Input: part model. Units: mm. Frame: model coordinates. Face numbers are marked on the shaded views. A direction names the side the tool comes from. Coordinates: 2 decimals unless noted, no trailing zeros. Order: outer loops, then holes, each group sorted by start corner. A loop starts at its lowest first (then second) coordinate and runs counter-clockwise, first axis right, second up. Notation, with made-up numbers: (8.25, 11) - (25.25, 11) arc R13 ccw to (25.25, 36) - close; hole circle Ø1 at (43, 22.5). An arc over 180 degrees is marked (long way). Answer as CSV lines item,"result". Start each with the question number.
Item 1: Draft query along Z for the marked faces 1, 2 and 3. Return one class per face: +Z half, -Z half, draft (parallel to the pull), parting line (faces both ways), or undercut.
Item 2: Section C-C (z = 14.25). Output: boundary loops of the cut face in (x, y), and give its area (3 significant figures).
Item 3: First-contact query: pin 1 (6 mm diameter, centred on x = -2, z = 11, fed in from -Y); pin 2 (1.6 mm diameter, centred on x = -3.5, z = 10.5, fed in from +Y); pin 3 (10 mm diameter, centred on y = 6, z = 9, fed in from -X); pin 4 (1.6 mm diameter, centred on x = -5, z = 10, fed in from -Y). Flat tips, straight axial feed; report the tip coordinate or a pass-through.
Item 4: Material intervals for line 1 along Z through (x, y) = (-3.25, 2.5); line 2 along Y through (x, z) = (-6.25, 10.5); line 3 along Z through (x, y) = (-6.5, 0.5), sorted ascending.
Item 5: Access query for the marked faces 4 and 5. Directions: +Z, -Z, +X, -X, +Y, -Y. A direction counts if a zero-diameter tool reaches every point of the face in a straight line with its end or side. Return the directions, or none.
Item 6: Section A-A (z = 9.75). Output: boundary loops of the cut face in (x, y).
Item 7: Section B-B (z = 7.5). Output: boundary loops of the cut face in (x, y), and give its area (3 significant figures).
Autodesk Fusion 360 part; units mm, degrees
sketch "Sketch1" plane through (0, 0, 0) normal (0, 0, 1) x (1, 0, 0)
  line L0 (0, 10) -> (0, -10)
  arc A0 (0, 10) -> (0, -10) centre (0, 0) ccw
extrude "Extrude1" add sketch "Sketch1" along normal blind 20
sketch "Sketch2" plane through (0, 0, 0) normal (1, 0, 0) x (0, 0, -1)
  line L0 (0, -10) -> (0, 10)
  line L1 (0, 10) -> (-20, 10)
  line L2 (-20, 10) -> (-20, -10)
  line L3 (-20, -10) -> (0, -10)
  line L4 (-8.4123, -2.75) -> (-6.8246, 0)
  line L5 (-6.8246, 0) -> (-8.4123, 2.75)
  line L6 (-8.4123, 2.75) -> (-11.5877, 2.75)
  line L7 (-11.5877, 2.75) -> (-13.1754, 0)
  line L8 (-13.1754, 0) -> (-11.5877, -2.75)
  line L9 (-11.5877, -2.75) -> (-8.4123, -2.75)
  point P0 (-10, 0)
  dimension "d3" = 2.75
extrude "Extrude2" cut sketch "Sketch2" against normal blind 7 contours L4 L5 L6 L7 L8 L9
chamfer "Chamfer1" distance 1 angle 45 6 edges at (0, 0, 20) (0, 10, 10) (0, -10, 10) (0, 0, 0) (-10, 0, 0) (-10, 0, 20)
equation "d3 = ( 5.5 / 2 ) * 1 mm"
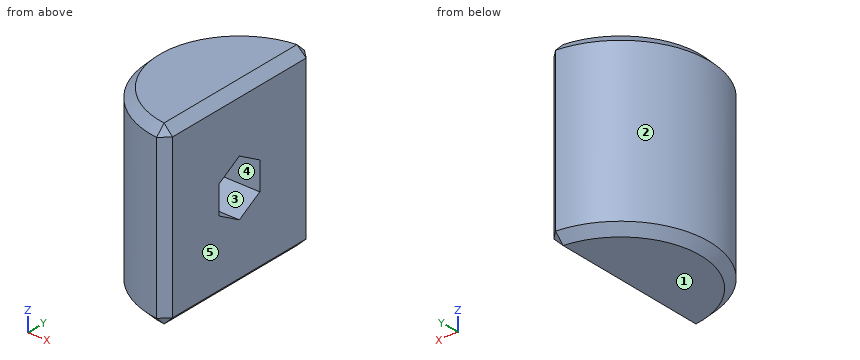
Determined:
1,face 1,"-Z half"
1,face 2,"draft"
1,face 3,"undercut"
2,outline,"(-1, -9.95) - (0, -9) - (0, 9) - (-1, 9.95) arc R10 ccw to start"
2,area,"156 mm^2"
3,pin 1,"stops at y = -9.95"
3,pin 2,"stops at y = 9.63"
3,pin 3,"stops at x = -9.95"
3,pin 4,"stops at y = -9.08"
4,line 1,"z = 0 to 8.27, 11.73 to 20"
4,line 2,"y = -7.81 to -2.75, 2.75 to 7.81"
4,line 3,"z = 0 to 7.11, 12.89 to 20"
5,face 4,"+X"
5,face 5,"+Z, -Z, +X, +Y, -Y"
6,outline,"(-7, -2.75) - (-7, 2.75) - (0, 2.75) - (0, 9) - (-1, 9.95) arc R10 ccw to (-1, -9.95) - (0, -9) - (0, -2.75) - close"
7,outline,"(-7, -1.17) - (-7, 1.17) - (0, 1.17) - (0, 9) - (-1, 9.95) arc R10 ccw to (-1, -9.95) - (0, -9) - (0, -1.17) - close"
7,area,"140 mm^2"
